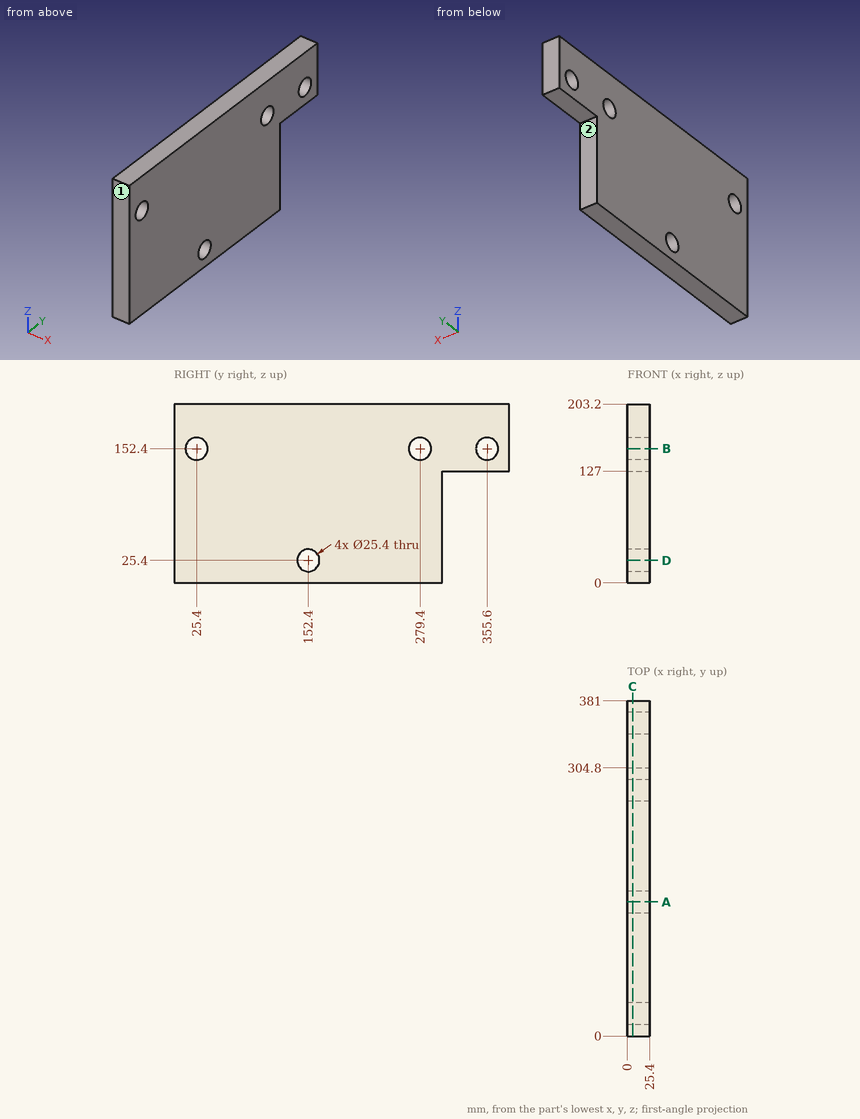
Input: dimensioned drawing with shaded views. Units: mm. Origin: part minimum x, y, z. A direction names the side the tool comes from. Give positions to 0.01 mm unless a question says otherwise; leave off trailing zeros. Write each loop counter-clockwise with the first axis right and the second up, starting at its lowest first coordinate (ties: lowest second). Pieces come first, ordered by that corner, then holes.
1. Section query B-B (z = 152.4). Return the cut outline in (x, y).
2. Section query C-C (x = 6). Return the cut outline in (y, z).
3. Section query D-D (z = 25.4). Return the cut outline in (x, y).
4. Access query for the marked faces 1 and 2. Directions: +Z, -Z, +X, -X, +Y, -Y. A direction counts if a zero-diameter tool reaches every point of the face in a straight line with its end or side. Return the directions, or none.
5. Section query A-A (y = 152.4). Return the cut outline in (x, z).
6. First-contact query: pin 1 (7.5 mm diameter, centred on x = 10.5, z = 52.5, fed in from +Y). Flat tip, straight axial feed; report the tip coordinate or a pass-through.
7. Material intervals for line 1 along Z through (x, y) = (7.5, 279.4); line 2 along Z through (x, y) = (17.25, 355.6); line 3 along Y through (x, z) = (9, 148), sorted ascending.
Output values:
1. outline: (0, 0) - (25.4, 0) - (25.4, 12.7) - (0, 12.7) - close; (0, 38.1) - (25.4, 38.1) - (25.4, 266.7) - (0, 266.7) - close; (0, 292.1) - (25.4, 292.1) - (25.4, 342.9) - (0, 342.9) - close; (0, 368.3) - (25.4, 368.3) - (25.4, 381) - (0, 381) - close
2. outline: (0, 0) - (304.8, 0) - (304.8, 127) - (381, 127) - (381, 203.2) - (0, 203.2) - close; hole circle Ø25.4 at (25.4, 152.4); hole circle Ø25.4 at (152.4, 25.4); hole circle Ø25.4 at (279.4, 152.4); hole circle Ø25.4 at (355.6, 152.4)
3. outline: (0, 0) - (25.4, 0) - (25.4, 139.7) - (0, 139.7) - close; (0, 165.1) - (25.4, 165.1) - (25.4, 304.8) - (0, 304.8) - close
4. face 1: +Z, -Z, +X, -X, -Y
4. face 2: -Z, +X, -X, +Y
5. outline: (0, 0) - (25.4, 0) - (25.4, 12.7) - (0, 12.7) - close; (0, 38.1) - (25.4, 38.1) - (25.4, 203.2) - (0, 203.2) - close
6. pin 1: stops at y = 304.8
7. line 1: z = 0 to 139.7, 165.1 to 203.2
7. line 2: z = 127 to 139.7, 165.1 to 203.2
7. line 3: y = 0 to 13.49, 37.31 to 267.49, 291.31 to 343.69, 367.51 to 381
